```python
from build123d import *

# Parameters (mm, degrees)
BASE_FLANGE1_DEPTH           = 2.65684
SKETCHED_BEND3_DEPTH         = 360.91368
SKETCHED_BEND3_2_DEPTH       = 360.91368
SKETCH10_R                   = 6.35
CUT_EXTRUDE2_DEPTH           = 2.65684
EDGE_FLANGE5_DEPTH           = 254
EDGE_FLANGE6_STRIP_W         = 16.97736
EDGE_FLANGE6_STRIP_H         = 2.65684
EDGE_FLANGE6_STRIP_CUT_DEPTH = 116.5225
EDGE_FLANGE6_DEPTH           = 116.5225
SKETCH36_R                   = 6.35
CUT_EXTRUDE3_DEPTH           = 2.65684


# Read off the part's stored shape, not the designer's step: Sketched Bend3
# Sheet-metal steps are written as plain solids
with BuildPart() as part:
    # Sketch1 → Base-Flange1 (new body)
    with BuildSketch(Plane.XY):
        with BuildLine():
            Line((0, 0), (0, 254))
            Line((0, 254), (167.75684, 254))
            ThreePointArc((167.75684, 254), (180.45684, 241.3), (193.15684, 254))
            Line((193.15684, 254), (360.91368, 254))
            Line((360.91368, 254), (360.91368, 0))
            Line((360.91368, 0), (360.91368, -57.15))
            Line((360.91368, -57.15), (0, -57.15))
            Line((0, -57.15), (0, 0))
        make_face()
    extrude(amount=-BASE_FLANGE1_DEPTH)

    # Sketched Bend3 outline → Sketched Bend3 (cut)
    with BuildSketch(Plane.YZ):
        with BuildLine():
            ThreePointArc((0, -2.65684), (-2.783367186, -1.949765838), (-4.891802611, 0))
            Line((-4.891802611, 0), (-57.15, 0))
            Line((-57.15, 0), (-57.15, -2.65684))
            Line((-57.15, -2.65684), (0, -2.65684))
        make_face()
    extrude(amount=SKETCHED_BEND3_DEPTH, mode=Mode.SUBTRACT)

    # Sketched Bend3 2 outline → Sketched Bend3 2 (add)
    with BuildSketch(Plane.YZ):
        with BuildLine():
            ThreePointArc((0, 0), (-2.24506403, 0.92993597), (-3.175, 3.175))
            Line((-3.175, 3.175), (-3.175, 53.251044406))
            Line((-3.175, 53.251044406), (-5.83184, 53.251044406))
            Line((-5.83184, 53.251044406), (-5.83184, 3.175))
            ThreePointArc((-5.83184, 3.175), (-5.591894488, 1.519381136), (-4.891802611, 0))
            Line((-4.891802611, 0), (0, 0))
        make_face()
    extrude(amount=SKETCHED_BEND3_2_DEPTH)

    # Sketch10 → Cut-Extrude2 (cut)
    with BuildSketch(Plane(origin=(0, -3.175, 0), x_dir=(1, 0, 0), z_dir=(0, 1, 0))):
        with Locations(Location((322.81368, -34.201044406, 0), (0, 0, 270))):
            Circle(SKETCH10_R)
        with Locations(Location((252.96368, -34.201044406, 0), (0, 0, 270))):
            Circle(SKETCH10_R)
        with Locations(Location((40.75684, -34.201044406, 0), (0, 0, 270))):
            Circle(SKETCH10_R)
        with Locations(Location((110.60684, -34.201044406, 0), (0, 0, 270))):
            Circle(SKETCH10_R)
        with Locations(Location((180.45684, -34.201044406, 0), (0, 0, 270))):
            Circle(SKETCH10_R)
    extrude(amount=-CUT_EXTRUDE2_DEPTH, mode=Mode.SUBTRACT)

    # Edge-Flange5 section (across the edge) → Edge-Flange5 (add)
    with BuildSketch(Plane(origin=(-3.175, 0, -2.65684), x_dir=(1, 0, 0), z_dir=(0, 1, 0))):
        with BuildLine():
            Line((-2.65684, 3.175), (-2.65684, 119.6975))
            Line((-2.65684, 119.6975), (0, 119.6975))
            Line((0, 119.6975), (0, 3.175))
            ThreePointArc((0, 3.175), (0.92993597, 0.92993597), (3.175, 0))
            Line((3.175, 0), (3.175, -2.65684))
            ThreePointArc((3.175, -2.65684), (-0.948733611, -0.948733611), (-2.65684, 3.175))
        make_face()
    extrude(amount=EDGE_FLANGE5_DEPTH)

    # Edge-Flange6 strip (across the edge) → Edge-Flange6 strip cut (cut)
    with BuildSketch(Plane(origin=(-5.83184, 254, -5.83184), x_dir=(0, -1, 0), z_dir=(0, 0, -1))):
        with Locations((-2.65684, -1.32842)):
            Rectangle(EDGE_FLANGE6_STRIP_W, EDGE_FLANGE6_STRIP_H)
    extrude(amount=EDGE_FLANGE6_STRIP_CUT_DEPTH, mode=Mode.SUBTRACT)

    # Edge-Flange6 section (across the edge) → Edge-Flange6 (add)
    with BuildSketch(Plane(origin=(-5.83184, 254, -5.83184), x_dir=(0, -1, 0), z_dir=(0, 0, -1))):
        with BuildLine():
            Line((0, 3.175), (0, 53.975))
            Line((0, 53.975), (2.65684, 53.975))
            Line((2.65684, 53.975), (2.65684, 3.175))
            ThreePointArc((2.65684, 3.175), (3.58677597, 0.92993597), (5.83184, 0))
            Line((5.83184, 0), (5.83184, -2.65684))
            ThreePointArc((5.83184, -2.65684), (1.708106389, -0.948733611), (0, 3.175))
        make_face()
    extrude(amount=EDGE_FLANGE6_DEPTH)

    # Sketch36 → Cut-Extrude3 (cut)
    with BuildSketch(Plane.ZY.offset(5.83184)):
        with Locations((-32.886251514, 45.966665125)):
            Circle(SKETCH36_R)
        with Locations((-89.021589499, 43.324159587)):
            Circle(SKETCH36_R)
    extrude(amount=-CUT_EXTRUDE3_DEPTH, mode=Mode.SUBTRACT)


solid = part.part
```
Check sheet for the modelled part. Datum: model origin and axes. Units: mm. A direction names the side the tool comes from. Coordinates: 2 decimals unless noted, no trailing zeros. Order: outer loops, then holes, each group sorted by start corner. A loop starts at its lowest first (then second) coordinate and runs counter-clockwise, first axis right, second up. Notation, with made-up numbers: M -35,84 L -17,84 A25 cw -17,101 Z; hole C -5.5,50 d3. An arc over 180 degrees is marked long. Write each question's results on one line, items separated by ' | '. Start each with the question number.
1. Cross-section at A-A on y = 204.5. Record the cut outline in (x, z) (3 decimals), and give its area (3 significant figures).
2. Cross-section at D-D on z = 19.5. Record the cut outline in (x, y) (3 decimals).
3. Cross-section at C-C on z = -105. Record the cut outline in (x, y) (3 decimals).
4. Access from +Z, -Z, +X, -X, +Y, -Y to the whole of each face (thin tool, end or side, straight path). Record for faces 1 (the face through (178, -3.175, 28)), 2 (the face through (-5.832, 122, -63)), 3 (the face through (183, 129, -2.657)), 4 (the face through (247.33, -4.48, 37.13)).
5. Cross-section at B-B on x = 293.5. Record the cut outline in (y, z) (3 decimals).
6. Go/stop test with flat-tipped pins: P1, Ø2, axis at x = 146, y = 85, coming from the +Z side; P2, Ø6, axis at x = 50.5, y = 206.5, coming from the -Z side; P3, Ø12, axis at x = -10.5, z = -30, coming from the -Y side. Record where each tip stops, or that it passes through.
7. Material ranges on probe 1 along Y at (x, z) = (126, 41) (3 decimals); probe 2 along Z at (x, y) = (33, 88), recorded low to high.
8. Mould release check, pull along Z, two halves, no side actions. Record for faces 5 (the face through (-35, 251.343, -63)), 6 (the face through (183, 129, 0)), 7 (the face through (115.961, -4.485, 37.615)): +Z half, -Z half, draft (parallel to the pull), parting line (faces both ways), or undercut.
Checks:
1) outline: M -5.832,-122.354 L -3.175,-122.354 L -3.175,-5.832 A3.175 cw 0,-2.657 L 360.914,-2.657 L 360.914,0 L 0,0 A5.832 ccw -5.832,-5.832 Z | area: 1,290 mm²
2) outline: M 0,-5.832 L 360.914,-5.832 L 360.914,-3.175 L 0,-3.175 Z
3) outline: M -59.807,251.343 L -9.007,251.343 A3.175 cw -5.832,248.168 L -5.832,0 L -3.175,0 L -3.175,248.168 A5.832 ccw -9.007,254 L -59.807,254 Z
4) face 1: +Z, +X, -X, +Y | face 2: +Z, -Z, -X, -Y | face 3: -Z, +X, +Y, -Y | face 4: +Y, -Y
5) outline: M -5.832,3.175 A5.832 ccw 0,-2.657 L 254,-2.657 L 254,0 L 0,0 A3.175 cw -3.175,3.175 L -3.175,53.251 L -5.832,53.251 Z
6) P1: stops at z = 0 | P2: stops at z = -2.66 | P3: stops at y = 0
7) probe 1: y = -5.832 to -3.175 | probe 2: z = -2.66 to 0
8) face 5: draft | face 6: +Z half | face 7: undercut
